Input: part model. Units: mm. Frame: model coordinates. A direction names the side the tool comes from. Round coordinates to 2 decimals unless told otherwise and drop trailing zeros. Loops run counter-clockwise (first coordinate to the right, second up) from the corner with the lowest first, then second, coordinate; pieces in that order, holes last. Notation, with made-up numbers: (79, 67.5) - (128, 67.5) arc R12 cw to (128, 81.5) - close; hole circle Ø10 at (-27, 59). An arc over 180 degrees is marked (long way). Use CSV: the item, a comma, the result in double quotes. Start each with the question number.
1. Cut plane A-A (x = 0). Return loops of the section in (y, z), and give its area (3 significant figures).
2. Cut plane C-C (x = 6). Return loops of the section in (y, z).
3. Cut plane D-D (z = 2.25). Give the number of separate pieces and of enclosed holes in the cut face, and give its area (3 significant figures).
4. Pin query (flat end, axial travel): P1, Ø1, axis at y = -7.5, z = -3, coming from the -X side; P2, Ø1.6, axis at x = 6, z = 0, coming from the +Y side; P3, Ø5, axis at x = -15.5, z = 0.5, coming from the +Y side. Return the tip coordinate at first contact, or that it passes through.
5. Access query for faces 4 (the cylindrical face through (14.6, -5.3, 0.1)), 5 (the flat face through (6, 22, 3)), 6 (the flat face through (-6, 16, 0)), 7 (the flat face through (22, -6, -3)). Directions: +Z, -Z, +X, -X, +Y, -Y. A direction counts if a zero-diameter tool reaches every point of the face in a straight line with its end or side. Return the directions, or none.
6. Material intervals for probe 1 along Z at (x, y) = (21.5, -6); probe 2 along X at (y, z) = (20, 4); probe 3 along X at (y, z) = (-5, 3.5) (3 decimals), sorted ascending. Write a range as from..to.
7. Pull-direction query (X, two-part tool) for faces 1 (the flat face through (4, 8, -5)), 2 (the flat face through (-16.849, -2.816, -0.014)), 3 (the flat face through (-23.02, -6.13, -3.99)); classes: +X half, -X half, draft (parallel to the pull), parting line (faces both ways), or undercut.
8. Cut plane B-B (y = 11). Return loops of the section in (x, z), and give its area (3 significant figures).
```python
from build123d import *

# Parameters (mm, degrees)
ESQUISSE1_R                  = 8
ESQUISSE1_R_2                = 1.25
BOSS_EXTRU_1_DEPTH           = 5
BOSS_EXTRU_1_DEPTH_BACK      = 5
ESQUISSE2_W                  = 6
ESQUISSE2_H                  = 2
ENL_V_MAT_EXTRU_1_DEPTH      = 19
ESQUISSE3_R                  = 1
ENL_V_MAT_EXTRU_2_DEPTH      = 5
R_P_TITION_CIRCULAIRE1_COUNT = 3
ESQUISSE5_R                  = 4
ENL_V_MAT_EXTRU_5_DEPTH      = 18


with BuildPart() as part:
    # Esquisse1 → Boss.-Extru.1 (new body, two sides)
    with BuildSketch(Plane.XY) as boss_extru_1_sk:
        with BuildLine():
            Line((24.668584287, -3.272758664), (21.418584287, -8.901923789))
            Line((21.418584287, -8.901923789), (15.356406461, -5.401923789))
            ThreePointArc((15.356406461, -5.401923789), (14.597587415, -5.302023366), (13.990381057, -5.767949192))
            Line((13.990381057, -5.767949192), (11.990381057, -9.232050808))
            ThreePointArc((11.990381057, -9.232050808), (11.890480634, -9.990869853), (12.356406461, -10.598076211))
            Line((12.356406461, -10.598076211), (18.418584287, -14.098076211))
            Line((18.418584287, -14.098076211), (15.168584287, -19.727241336))
            Line((15.168584287, -19.727241336), (2, -12.124355653))
            ThreePointArc((2, -12.124355653), (0, -11.588457268), (-2, -12.124355653))
            Line((-2, -12.124355653), (-15.168584287, -19.727241336))
            Line((-15.168584287, -19.727241336), (-18.418584287, -14.098076211))
            Line((-18.418584287, -14.098076211), (-12.356406461, -10.598076211))
            ThreePointArc((-12.356406461, -10.598076211), (-11.890480634, -9.990869853), (-11.990381057, -9.232050808))
            Line((-11.990381057, -9.232050808), (-13.990381057, -5.767949192))
            ThreePointArc((-13.990381057, -5.767949192), (-14.597587415, -5.302023366), (-15.356406461, -5.401923789))
            Line((-15.356406461, -5.401923789), (-21.418584287, -8.901923789))
            Line((-21.418584287, -8.901923789), (-24.668584287, -3.272758664))
            Line((-24.668584287, -3.272758664), (-11.5, 4.330127019))
            ThreePointArc((-11.5, 4.330127019), (-10.035898385, 5.794228634), (-9.5, 7.794228634))
            Line((-9.5, 7.794228634), (-9.5, 23))
            Line((-9.5, 23), (-3, 23))
            Line((-3, 23), (-3, 16))
            ThreePointArc((-3, 16), (-2.707106781, 15.292893219), (-2, 15))
            Line((-2, 15), (2, 15))
            ThreePointArc((2, 15), (2.707106781, 15.292893219), (3, 16))
            Line((3, 16), (3, 23))
            Line((3, 23), (9.5, 23))
            Line((9.5, 23), (9.5, 7.794228634))
            ThreePointArc((9.5, 7.794228634), (10.035898385, 5.794228634), (11.5, 4.330127019))
            Line((11.5, 4.330127019), (24.668584287, -3.272758664))
        make_face()
        Circle(ESQUISSE1_R, mode=Mode.SUBTRACT)
        with Locations((0, 11)):
            Circle(ESQUISSE1_R_2, mode=Mode.SUBTRACT)
        with Locations((9.526279442, -5.5)):
            Circle(ESQUISSE1_R_2, mode=Mode.SUBTRACT)
        with Locations((-9.526279442, -5.5)):
            Circle(ESQUISSE1_R_2, mode=Mode.SUBTRACT)
    extrude(amount=BOSS_EXTRU_1_DEPTH)
    extrude(boss_extru_1_sk.sketch, amount=-BOSS_EXTRU_1_DEPTH_BACK)

    # Esquisse2 → Enl_v. mat.-Extru.1 (cut)
    with BuildSketch(Plane.ZY.offset(9.5)):
        with Locations((0, 22)):
            Rectangle(ESQUISSE2_W, ESQUISSE2_H)
    enl_v_mat_extru_1 = extrude(amount=-ENL_V_MAT_EXTRU_1_DEPTH, mode=Mode.SUBTRACT)

    # Esquisse3 → Enl_v. mat.-Extru.2 (cut)
    with BuildSketch(Plane(origin=(0, 21, 0), x_dir=(1, 0, 0), z_dir=(0, 1, 0))):
        with Locations((-6, 0)):
            Circle(ESQUISSE3_R)
        with Locations((6, 0)):
            Circle(ESQUISSE3_R)
    enl_v_mat_extru_2 = extrude(amount=-ENL_V_MAT_EXTRU_2_DEPTH, mode=Mode.SUBTRACT)

    # R_p_tition circulaire1: Enl_v. mat.-Extru.1, Enl_v. mat.-Extru.2 ×3 about axis
    r_p_tition_circulaire1_axis = Axis((0, 0, 0), (0, 0, 1))
    for i in range(1, R_P_TITION_CIRCULAIRE1_COUNT):
        add(enl_v_mat_extru_1.rotate(r_p_tition_circulaire1_axis, i * 360 / R_P_TITION_CIRCULAIRE1_COUNT), mode=Mode.SUBTRACT)
        add(enl_v_mat_extru_2.rotate(r_p_tition_circulaire1_axis, i * 360 / R_P_TITION_CIRCULAIRE1_COUNT), mode=Mode.SUBTRACT)

    # Esquisse5 → Enl_v. mat.-Extru.5 (cut)
    with BuildSketch(Plane(origin=(0, 0, 0), x_dir=(1, 0, 0), z_dir=(0, 1, 0))):
        Circle(ESQUISSE5_R)
    extrude(amount=-ENL_V_MAT_EXTRU_5_DEPTH, mode=Mode.SUBTRACT)


solid = part.part
```
Established:
1,outline,"(-11.59, -5) - (-8, -5) - (-8, -4) - (-11.59, -4) - close; (-11.59, 4) - (-8, 4) - (-8, 5) - (-11.59, 5) - close; (8, -5) - (9.75, -5) - (9.75, 5) - (8, 5) - close; (12.25, -5) - (15, -5) - (15, 5) - (12.25, 5) - close"
1,area,"52.2 mm2"
2,outline,"(-14.43, -5) - (-5.29, -5) - (-5.29, 5) - (-14.43, 5) - close; (5.29, -5) - (23, -5) - (23, -3) - (21, -3) - (21, -1) - (16, -1) - (16, 1) - (21, 1) - (21, 3) - (23, 3) - (23, 5) - (5.29, 5) - close"
3,separate pieces,"1"
3,enclosed holes,"3"
3,area,"692 mm2"
4,P1,"stops at x = -22.52"
4,P2,"stops at y = 16"
4,P3,"stops at y = 3.46"
5,face 4,"+Z, -Z"
5,face 5,"+X, -X, +Y"
5,face 6,"+Y"
5,face 7,"+X, -Y"
6,probe 1,"z = -5..-3, 3..5"
6,probe 2,"x = -9.5..-3, 3..9.5"
6,probe 3,"x = -23.671..-10.672, -8.381..-6.245, 6.245..8.381, 10.672..23.671"
7,face 1,"draft"
7,face 2,"undercut"
7,face 3,"-X half"
8,outline,"(-9.5, -5) - (-1.25, -5) - (-1.25, 5) - (-9.5, 5) - close; (1.25, -5) - (9.5, -5) - (9.5, 5) - (1.25, 5) - close"
8,area,"165 mm2"
